```python
from build123d import *

# Parameters (mm, degrees)
SKETCH1_W           = 16
SKETCH1_H           = 90
SKETCH1_R           = 2.2
BOSS_EXTRUDE1_DEPTH = 28
SKETCH2_W           = 23
SKETCH2_H           = 58
CUT_EXTRUDE1_DEPTH  = 16
SKETCH3_R           = 4
CUT_EXTRUDE2_DEPTH  = 22
FILLET1_R           = 2


with BuildPart() as part:
    # Sketch1 → Boss-Extrude1 (new body)
    with BuildSketch(Plane.XY):
        with Locations((8, 45)):
            Rectangle(SKETCH1_W, SKETCH1_H)
        with Locations((8, 82)):
            Circle(SKETCH1_R, mode=Mode.SUBTRACT)
        with Locations((8, 8)):
            Circle(SKETCH1_R, mode=Mode.SUBTRACT)
    extrude(amount=BOSS_EXTRUDE1_DEPTH)

    # Sketch2 → Cut-Extrude1 (cut)
    with BuildSketch(Plane(origin=(16, 0, 0), x_dir=(0, 0, -1), z_dir=(1, 0, 0))):
        with Locations((-11.5, 45)):
            Rectangle(SKETCH2_W, SKETCH2_H)
    extrude(amount=-CUT_EXTRUDE1_DEPTH, mode=Mode.SUBTRACT)

    # Sketch3 → Cut-Extrude2 (cut)
    with BuildSketch(Plane.XY.offset(28)):
        with Locations((8, 82)):
            Circle(SKETCH3_R)
        with Locations((8, 8)):
            Circle(SKETCH3_R)
    extrude(amount=-CUT_EXTRUDE2_DEPTH, mode=Mode.SUBTRACT)

    # Fillet1
    fillet1_edges = [part.edges().sort_by_distance(p)[0] for p in [
        (16, 45, 28),
        (8, 90, 28),
        (16, 74, 11.5),
        (16, 45, 23),
        (16, 16, 11.5),
        (0, 16, 11.5),
        (0, 45, 23),
        (0, 74, 11.5),
        (0, 45, 28),
        (0, 90, 14),
        (16, 90, 14),
        (16, 0, 14),
        (0, 0, 14),
        (8, 0, 28),
    ]]
    fillet(fillet1_edges, radius=FILLET1_R)


solid = part.part
```
Part model, mm, in its own coordinate system. A direction names the side the tool comes from. Give positions to 0.01 mm unless a question says otherwise; leave off trailing zeros. Loops run counter-clockwise (first coordinate to the right, second up) from the corner with the lowest first, then second, coordinate; pieces in that order, holes last. Notation, with made-up numbers: M 16,25 L 20,25 A13 ccw 20,34 Z; hole C -15,48.25 d3. An arc over 180 degrees is marked long. Return JSON: item names as keys, results as strings.
1) Saw through at A-A, the plane z = 11. List the corners of the cut face in (x, y).
Calculated:
{"outline": "M 0,2 A2 ccw 2,0 L 14,0 A2 ccw 16,2 L 16,14 A2 ccw 14,16 L 2,16 A2 ccw 0,14 Z; M 0,76 A2 ccw 2,74 L 14,74 A2 ccw 16,76 L 16,88 A2 ccw 14,90 L 2,90 A2 ccw 0,88 Z; hole C 8,8 d8; hole C 8,82 d8"}
2) Pull direction Y, two halves, no side cores. Call faces 1 (the face through (0.57, 0.6, 13.18)), 2 (the face through (0.57, 74.6, 12.32)), 3 (the face through (0, 48, 25.5)): released by +Y, released by -Y, zero draft, split by the parting line, or undercut.
Calculated:
{"face 1": "released by -Y", "face 2": "undercut", "face 3": "zero draft"}
3) Saw through at D-D, the plane y = 50. List the corners of the cut face in (x, z).
Calculated:
{"outline": "M 0,25 A2 ccw 2,23 L 14,23 A2 ccw 16,25 L 16,26 A2 ccw 14,28 L 2,28 A2 ccw 0,26 Z"}
4) 3-axis set-ups, long thin cutter, end or side, ignore diameter. For faces 4 (the face through (0.57, 45.43, 23.6)), 5 (the face through (8, 16, 12)), 6 (the face through (15.4, 74.57, 12.32)), 7 (the face through (15.4, 45.6, 27.43)), 8 (the face through (7.133, 78.095, 17.154)): which of +Z, -Z, +X, -X, +Y, -Y reach the whole face in a straight line?
Calculated:
{"face 4": "-Z, -X", "face 5": "-Z, +X, -X", "face 6": "-Z, +X", "face 7": "+Z, +X, +Y, -Y", "face 8": "+Z"}
5) Drill centre lines: line 1 (Y direction, x = 8, z = 2); line 2 (Y direction, x = 7.75, z = 14); line 3 (Y direction, x = 7.75, z = 24). Where is each one in solid material? Low to high.
Calculated:
{"line 1": "y = 0 to 5.8, 10.2 to 16, 74 to 79.8, 84.2 to 90", "line 2": "y = 0 to 4.01, 11.99 to 16, 74 to 78.01, 85.99 to 90", "line 3": "y = 0 to 4.01, 11.99 to 78.01, 85.99 to 90"}
6) Saw through at C-C, the plane x = 8. List the corners of the cut face in (y, z), then the cut area to 3 significant figures.
Calculated:
{"outline": "M 0,0 L 5.8,0 L 5.8,6 L 4,6 L 4,28 L 2,28 A2 ccw 0,26 Z; M 10.2,0 L 16,0 L 16,23 L 74,23 L 74,0 L 79.8,0 L 79.8,6 L 78,6 L 78,28 L 12,28 L 12,6 L 10.2,6 Z; M 84.2,0 L 90,0 L 90,26 A2 ccw 88,28 L 86,28 L 86,6 L 84.2,6 Z", "area": "779 mm2"}
7) Saw through at B-B, the plane y = 8. List the corners of the cut face in (x, z).
Calculated:
{"outline": "M 0,0 L 5.8,0 L 5.8,6 L 4,6 L 4,28 L 2,28 A2 ccw 0,26 Z; M 10.2,0 L 16,0 L 16,26 A2 ccw 14,28 L 12,28 L 12,6 L 10.2,6 Z"}
8) Flat gauge pins, fed straight in: pin 1 Ø2.5 at (x, y) = (8, 8) entering from -Z; pin 2 Ø4 at (x, y) = (9, 9) entering from +Z; pin 3 Ø5 at (x, y) = (9.5, 65) entering from -Z. Where does each tip first touch, or does it go through?
Calculated:
{"pin 1": "passes through", "pin 2": "stops at z = 6", "pin 3": "stops at z = 23"}
